from build123d import *

# Parameters (mm, degrees)
SKETCH1_R           = 11.938
SKETCH1_R_2         = 8.763
BOSS_EXTRUDE1_DEPTH = 5.08
SKETCH2_R           = 11.938
BOSS_EXTRUDE2_DEPTH = 2.54
BOSS_EXTRUDE4_DEPTH = 2.54


with BuildPart() as part:
    # Sketch1 → Boss-Extrude1 (new body)
    with BuildSketch(Plane.XY):
        Circle(SKETCH1_R)
        Circle(SKETCH1_R_2, mode=Mode.SUBTRACT)
    extrude(amount=BOSS_EXTRUDE1_DEPTH)

    # Sketch2 → Boss-Extrude2 (add)
    with BuildSketch(Plane.XY.offset(5.08)):
        Circle(SKETCH2_R)
    extrude(amount=BOSS_EXTRUDE2_DEPTH)

    # Sketch3 → Boss-Extrude4 (add)
    with BuildSketch(Plane.XY.offset(7.62)):
        with BuildLine():
            Line((-3.643894956, -4.288673329), (-3.643894956, -3.805293576))
            ThreePointArc((-3.643894956, -3.805293576), (-2.21771863, -1.200372389), (-1.871410538, 1.749146896))
            Line((-1.871410538, 1.749146896), (-3.079634877, 1.749146896))
            Line((-3.079634877, 1.749146896), (-3.079634877, 3.601746254))
            Line((-3.079634877, 3.601746254), (-2.425208939, 3.601746254))
            ThreePointArc((-2.425208939, 3.601746254), (-2.683961488, 5.381731454), (-1.744311698, 6.915471479))
            Line((-1.744311698, 6.915471479), (-1.242224022, 6.915471479))
            Line((-1.242224022, 6.915471479), (-1.242224022, 4.985805442))
            Line((-1.242224022, 4.985805442), (-0.906720977, 4.849479664))
            Line((-0.906720977, 4.849479664), (-0.906720977, 7.372630859))
            Line((-0.906720977, 7.372630859), (-0.805595188, 7.372630859))
            ThreePointArc((-0.805595188, 7.372630859), (0.04512934, 8.694352218), (0.760232512, 7.294599731))
            ThreePointArc((0.760232512, 7.294599731), (2.43882488, 5.829651294), (2.425208939, 3.601746254))
            Line((2.425208939, 3.601746254), (3.079634877, 3.601746254))
            Line((3.079634877, 3.601746254), (3.079634877, 1.749146896))
            Line((3.079634877, 1.749146896), (1.871410538, 1.749146896))
            ThreePointArc((1.871410538, 1.749146896), (2.21771863, -1.200372389), (3.643894956, -3.805293576))
            Line((3.643894956, -3.805293576), (3.643894956, -4.288673329))
            Line((3.643894956, -4.288673329), (4.180733459, -4.288673329))
            Line((4.180733459, -4.288673329), (4.180733459, -6.661736262))
            Line((4.180733459, -6.661736262), (-4.235077354, -6.661736262))
            Line((-4.235077354, -6.661736262), (-4.235077354, -4.288673329))
            Line((-4.235077354, -4.288673329), (-3.643894956, -4.288673329))
        make_face()
    extrude(amount=BOSS_EXTRUDE4_DEPTH)


solid = part.part
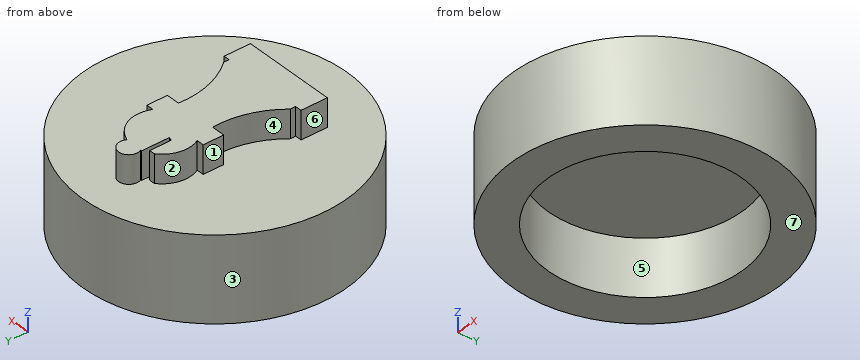
The listing builds one solid part. Answer for the finished solid, in the listing's coordinates (mm). Face numbers are marked on the shaded views. A direction names the side the tool comes from. Give positions to 0.01 mm unless a question says otherwise; leave off trailing zeros. Write each loop counter-clockwise with the first axis right and the second up, starting at its lowest first coordinate (ties: lowest second). Pieces come first, ordered by that corner, then holes.
1) Section A-A (x = 0) is taken. Write down the section's boundary in (y, z).
2) For a pull along Y with two mould halves and no side action, classify the marked faces 1, 2, 3 and 4 as pulls with the +Y half, pulls with the -Y half, needs draft (parallel to the pull), parting line crosses it, or undercut.
3) Find the intervals of material crossed by L1, parallel to Y at x = 0, z = 1.4; L2, parallel to Z at x = -8, y = -6.25; L3, parallel to Z at x = 2, y = -4.5, in increasing order.
4) Section C-C (y = 5.75) is taken. Write down the section's boundary in (x, z).
5) Section B-B (z = 2.5) is taken. Write down the section's boundary in (x, y).
6) Given P1, Ø1, axis at x = -7.5, y = -8.5, coming from the -Z side; P2, Ø1.3, axis at y = 6, z = 9.5, coming from the -X side; P3, Ø1.2, axis at y = -5, z = 9, coming from the +X side; P4, Ø1.3, axis at x = 2.5, z = 9.5, coming from the -Y side, each flat-ended and moving along its own axis, determine where each tip first touches the part or whether it passes through.
7) Section D-D (z = 8.75) is taken. Write down the section's boundary in (x, y).
8) A tool of negligible diameter and unlimited length cuts with its end or side. For the marked faces 5, 6 and 7, from which of +Z, -Z, +X, -X, +Y, -Y can it reach the whole face along a straight path? Write none if from no direction.
Response:
1. outline: (-11.94, 0) - (-8.76, 0) - (-8.76, 5.08) - (8.76, 5.08) - (8.76, 0) - (11.94, 0) - (11.94, 7.62) - (8.7, 7.62) - (8.7, 10.16) - (-6.66, 10.16) - (-6.66, 7.62) - (-11.94, 7.62) - close
2. face 1: needs draft
2. face 2: undercut
2. face 3: parting line crosses it
2. face 4: undercut
3. L1: y = -11.94 to -8.76, 8.76 to 11.94
3. L2: z = 0 to 7.62
3. L3: z = 5.08 to 10.16
4. outline: (-10.46, 0) - (-6.61, 0) - (-6.61, 5.08) - (6.61, 5.08) - (6.61, 0) - (10.46, 0) - (10.46, 7.62) - (2.47, 7.62) - (2.47, 10.16) - (-0.91, 10.16) - (-0.91, 7.62) - (-1.24, 7.62) - (-1.24, 10.16) - (-2.58, 10.16) - (-2.58, 7.62) - (-10.46, 7.62) - close
5. outline: circle Ø23.88 at (0, 0); hole circle Ø17.53 at (0, 0)
6. P1: stops at z = 0
6. P2: stops at x = -2.69
6. P3: stops at x = 4.18
6. P4: stops at y = -6.66
7. outline: (-4.24, -6.66) - (4.18, -6.66) - (4.18, -4.29) - (3.64, -4.29) - (3.64, -3.81) arc R7.78 cw to (1.87, 1.75) - (3.08, 1.75) - (3.08, 3.6) - (2.43, 3.6) arc R2.67 ccw to (0.76, 7.29) arc R0.91 ccw (long way) to (-0.81, 7.37) - (-0.91, 7.37) - (-0.91, 4.85) - (-1.24, 4.99) - (-1.24, 6.92) - (-1.74, 6.92) arc R2.64 ccw to (-2.43, 3.6) - (-3.08, 3.6) - (-3.08, 1.75) - (-1.87, 1.75) arc R7.78 cw to (-3.64, -3.81) - (-3.64, -4.29) - (-4.24, -4.29) - close
8. face 5: -Z
8. face 6: +Z, -X, +Y, -Y
8. face 7: -Z, +X, -X, +Y, -Y
